Input: part model. Units: mm. Frame: model coordinates. A direction names the side the tool comes from. Coordinates: 2 decimals unless noted, no trailing zeros. Write each loop counter-clockwise with the first axis right and the second up, starting at its lowest first coordinate (ties: lowest second). Pieces come first, ordered by that corner, then holes. Notation, with made-up numbers: M -11.75,85.5 L 19.25,85.5 A11 ccw 19.25,93.5 Z; hole C 11.25,63.25 d8. An arc over 180 degrees is marked long. Use one line per item in the form item = value.
from build123d import *

# Parameters (mm, degrees)
F0_R     = 12.7
F0_R_2   = 9.525
F0_R_3   = 6.35
F1_DEPTH = 6.35
F2_R     = 13.97
F3_DEPTH = 2.54


with BuildPart() as f1:
    # F0 (on Top) → F1 (new body, symmetric)
    with BuildSketch(Plane.XY):
        with BuildLine():
            Line((3.379315, 43.545812), (-16.448267, 9.610256))
            ThreePointArc((-16.448267, 9.610256), (-16.522377, -9.482276), (0, -19.05))
            Line((0, -19.05), (88.9, -19.05))
            ThreePointArc((88.9, -19.05), (102.841054, -5.978839), (90.693954, 8.774336))
            ThreePointArc((90.693954, 8.774336), (52.435987, 20.825014), (20.697055, 45.351147))
            ThreePointArc((20.697055, 45.351147), (11.580711, 48.836816), (3.379315, 43.545812))
        make_face()
        Circle(F0_R, mode=Mode.SUBTRACT)
        with Locations((88.9, -5.08)):
            Circle(F0_R_2, mode=Mode.SUBTRACT)
        with Locations((12.7, 38.1)):
            Circle(F0_R_3, mode=Mode.SUBTRACT)
    extrude(amount=F1_DEPTH, both=True)

    # F2 (on face) → F3 (cut)
    with BuildSketch(Plane.XY.offset(6.35)):
        Circle(F2_R)
    extrude(amount=-F3_DEPTH, mode=Mode.SUBTRACT)


solid = f1.part
(1) Section query C-C on x = 85. Return the cut outline in (y, z).
Computed:
outline = M -19.05,-6.35 L -13.77,-6.35 L -13.77,6.35 L -19.05,6.35 Z; M 3.61,-6.35 L 9.66,-6.35 L 9.66,6.35 L 3.61,6.35 Z
(2) Pull-direction query (Y, two-part tool) for faces 1 (the flat face through (28, 8, -6.35)), 2 (the cylindrical face through (-2.75, -12.4, -1.34)), 3 (the cylindrical face through (52.937, 20.565, 0.089)); classes: pulls with the +Y half, pulls with the -Y half, needs draft (parallel to the pull), parting line crosses it, or undercut.
Computed:
face_1 = needs draft
face_2 = undercut
face_3 = pulls with the +Y half
(3) First-contact query: pin 1 Ø8.5 at (x, y) = (5.5, 5) entering from +Z. Flat tip, straight axial feed; report the tip coordinate or a pass-through.
Computed:
pin_1 = through
(4) Line query: probe 1 along X at (y, z) = (-6, 0); probe 2 along X at (y, z) = (0, -1); probe 3 along Y at (x, z) = (88.9, -2.75) (3 decimals). Output: solid intervals per line, ascending.
Computed:
probe_1 = -18.08 to -11.19, 11.19 to 79.42, 98.38 to 102.84
probe_2 = -19.05 to -12.7, 12.7 to 80.84, 96.96 to 101.91
probe_3 = -19.05 to -14.605, 4.445 to 9.021
(5) Section query B-B on y = 2.5. Return the cut outline in (x, z).
Computed:
outline = M -18.89,-6.35 L -12.45,-6.35 L -12.45,3.81 L -13.74,3.81 L -13.74,6.35 L -18.89,6.35 Z; M 12.45,-6.35 L 83.13,-6.35 L 83.13,6.35 L 13.74,6.35 L 13.74,3.81 L 12.45,3.81 Z; M 94.67,-6.35 L 100.63,-6.35 L 100.63,6.35 L 94.67,6.35 Z
(6) Section query D-D on y = 42. Return the cut outline in (x, z).
Computed:
outline = M 2.48,-6.35 L 7.69,-6.35 L 7.69,6.35 L 2.48,6.35 Z; M 17.71,-6.35 L 23.86,-6.35 L 23.86,6.35 L 17.71,6.35 Z
(7) Section query A-A on z = 2. Return the cut outline in (x, y) (3 decimals), plus the area to 3 significant figures.
Computed:
outline = M -16.448,9.61 A19.05 ccw 0,-19.05 L 88.9,-19.05 A13.97 ccw 90.694,8.774 A114.3 cw 20.697,45.351 A10.795 ccw 3.379,43.546 Z; hole C 0,0 d25.4; hole C 12.7,38.1 d12.7; hole C 88.9,-5.08 d19.05
area = 4,240 mm^2
(8) Set-up query: faces 4 (the cylindrical face through (-1.82, 13.85, 5.1)), 5 (the cylindrical face through (102.82, -6.27, 0.09)). Return all of +Z, -Z, +X, -X, +Y, -Y with unobstructed straight access to the full face (end or side cutting, diameter ignored); none if empty.
Computed:
face_4 = +Z
face_5 = +Z, -Z, +X
